Geometry: see drawing. Coordinates: mm, zero at the bounding-box minimum. A direction names the side the tool comes from. Give positions to 0.01 mm unless a question says otherwise; leave off trailing zeros. Loops run counter-clockwise (first coordinate to the right, second up) from the corner with the lowest first, then second, coordinate; pieces in that order, holes last. Notation, with made-up numbers: (65, -27) -> (90, -27) arc R23 ccw to (90, -1) -> close; hole circle Ø1 at (53.5, 34). An arc over 180 degrees is marked (long way). Return JSON: item names as keys, results as strings. Group by question number.
(1) Cut plane C-C on x = 16.5. Return loops of the section in (y, z), then the cut area to 3 significant figures.
(2) Access query for the marked faces 5 and 6. Directions: +Z, -Z, +X, -X, +Y, -Y. A direction counts if a zero-diameter tool reaches every point of the face in a straight line with its end or side. Return the directions, or none.
(3) Cut plane A-A on y = 2.5. Return loops of the section in (x, z).
(4) Draft query along Z for the marked faces 1, 2, 3 and 4. Return one class per face: released by +Z, released by -Z, zero draft, split by the parting line, or undercut.
(5) Cut plane D-D on z = 27. Return loops of the section in (x, y), then the cut area to 3 significant figures.
(6) Cut plane B-B on z = 16.5. Return loops of the section in (x, y).
(7) Ray query, line 1 (Z direction, x = 9.5, y = 1.05); line 2 (X direction, y = 2.7, z = 12.5). Return the intervals inside material, ascending. Write a range as from..to.
(8) Pin query (flat end, axial travel): pin 1 (14 mm diameter, centred on x = 16.5, z = 16.5, fed in from -Y); pin 2 (2 mm diameter, centred on x = 5.5, z = 16, fed in from -Y). Return the tip coordinate at first contact, or that it passes through.
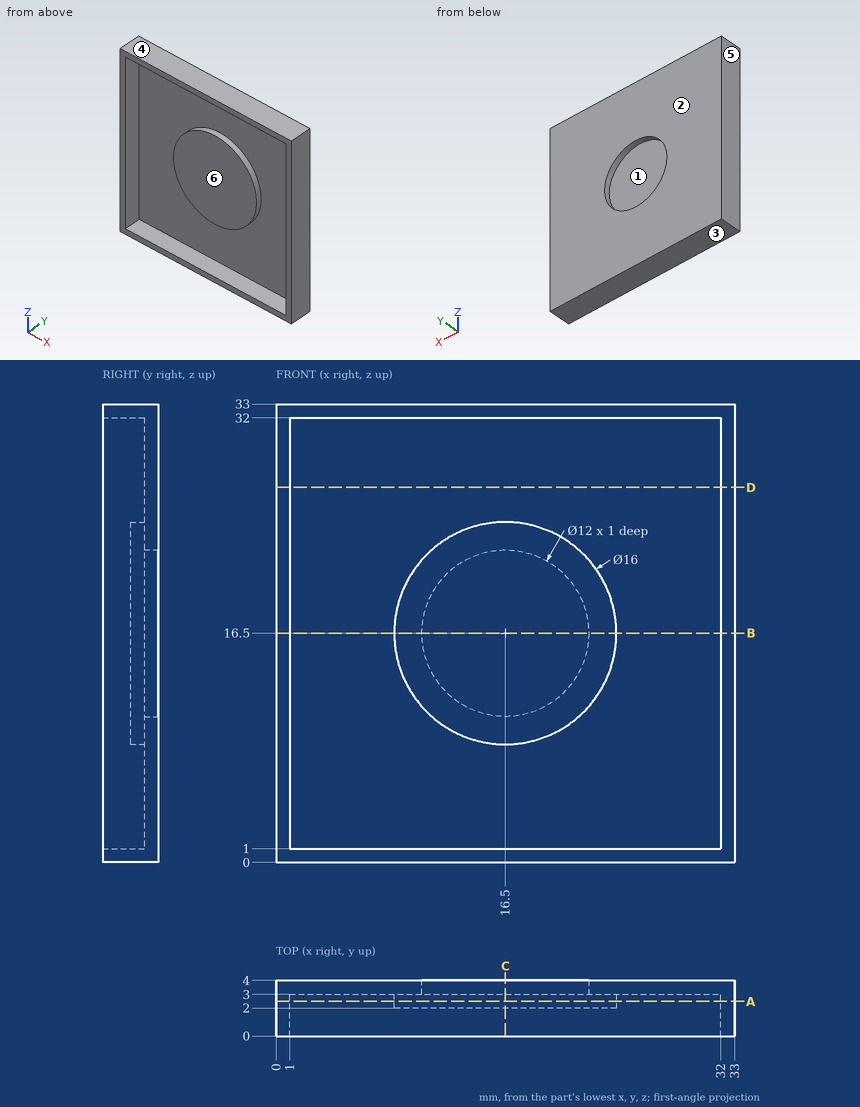
Answers:
{
 "1": {"outline": "(0, 0) -> (4, 0) -> (4, 10.5) -> (3, 10.5) -> (3, 22.5) -> (4, 22.5) -> (4, 33) -> (0, 33) -> (0, 32) -> (3, 32) -> (3, 24.5) -> (2, 24.5) -> (2, 8.5) -> (3, 8.5) -> (3, 1) -> (0, 1) -> close", "area": "43.0 mm²"},
 "2": {"face 5": "+Z, -Z, -X, +Y, -Y", "face 6": "-Y"},
 "3": {"outline": "(0, 0) -> (33, 0) -> (33, 33) -> (0, 33) -> close; circle Ø16 at (16.5, 16.5); hole (1, 1) -> (32, 1) -> (32, 32) -> (1, 32) -> close"},
 "4": {"face 1": "undercut", "face 2": "zero draft", "face 3": "released by -Z", "face 4": "released by +Z"},
 "5": {"outline": "(0, 0) -> (1, 0) -> (1, 3) -> (32, 3) -> (32, 0) -> (33, 0) -> (33, 4) -> (0, 4) -> close", "area": "39.0 mm²"},
 "6": {"outline": "(0, 0) -> (1, 0) -> (1, 3) -> (8.5, 3) -> (8.5, 2) -> (24.5, 2) -> (24.5, 3) -> (32, 3) -> (32, 0) -> (33, 0) -> (33, 4) -> (22.5, 4) -> (22.5, 3) -> (10.5, 3) -> (10.5, 4) -> (0, 4) -> close"},
 "7": {"line 1": "0..1, 32..33", "line 2": "0..1, 9.57..23.43, 32..33"},
 "8": {"pin 1": "y = 2", "pin 2": "y = 3"}
}
